```python
from build123d import *

# Parameters (mm, degrees)
SKETCH1_R           = 2.0701
SKETCH1_R_2         = 14.2875
BOSS_EXTRUDE1_DEPTH = 2.286


with BuildPart() as part:
    # Sketch1 → Boss-Extrude1 (new body)
    with BuildSketch(Plane.XY.offset(2.286)):
        with BuildLine():
            Line((-24.282138093, -1.253612903), (-13.20363246, -27.386969147))
            ThreePointArc((-13.20363246, -27.386969147), (-12.827181753, -28.600844397), (-12.7, -29.865373188))
            Line((-12.7, -29.865373188), (-12.7, -65.148356459))
            Line((-12.7, -65.148356459), (-11.173356459, -66.675))
            Line((-11.173356459, -66.675), (11.173356459, -66.675))
            Line((11.173356459, -66.675), (12.7, -65.148356459))
            Line((12.7, -65.148356459), (12.7, -29.865373188))
            ThreePointArc((12.7, -29.865373188), (12.827181753, -28.600844397), (13.20363246, -27.386969147))
            Line((13.20363246, -27.386969147), (24.282138093, -1.253612903))
            Line((24.282138093, -1.253612903), (24.282138093, 0.905387097))
            Line((24.282138093, 0.905387097), (13.596092395, 19.110856459))
            Line((13.596092395, 19.110856459), (12.069448854, 20.6375))
            Line((12.069448854, 20.6375), (-12.069448854, 20.6375))
            Line((-12.069448854, 20.6375), (-13.596092395, 19.110856459))
            Line((-13.596092395, 19.110856459), (-24.282138093, 0.905387097))
            Line((-24.282138093, 0.905387097), (-24.282138093, -1.253612903))
        make_face()
        with Locations((-9.2075, 15.947857811)):
            Circle(SKETCH1_R, mode=Mode.SUBTRACT)
        with Locations((-18.415, 0)):
            Circle(SKETCH1_R, mode=Mode.SUBTRACT)
        with Locations((0, -47.625)):
            Circle(SKETCH1_R, mode=Mode.SUBTRACT)
        with Locations((0, -22.225)):
            Circle(SKETCH1_R, mode=Mode.SUBTRACT)
        Circle(SKETCH1_R_2, mode=Mode.SUBTRACT)
        with Locations((0, -34.925)):
            Circle(SKETCH1_R, mode=Mode.SUBTRACT)
        with Locations((0, -60.325)):
            Circle(SKETCH1_R, mode=Mode.SUBTRACT)
        with Locations((18.415, 0)):
            Circle(SKETCH1_R, mode=Mode.SUBTRACT)
        with Locations((9.2075, 15.947857811)):
            Circle(SKETCH1_R, mode=Mode.SUBTRACT)
    extrude(amount=-BOSS_EXTRUDE1_DEPTH)


solid = part.part
```
CAD build for the part. Positions are in the model's coordinates, mm. A direction names the side the tool comes from. Coordinates: 2 decimals unless noted, no trailing zeros. Order: outer loops, then holes, each group sorted by start corner. A loop starts at its lowest first (then second) coordinate and runs counter-clockwise, first axis right, second up. Notation, with made-up numbers: (43.25, 32) - (90.25, 32) arc R33 cw to (90.25, 63) - close; hole circle Ø4 at (39, -36). An arc over 180 degrees is marked (long way). Answer in a Markdown table with one row per item.
1. 3-axis set-ups, long thin cutter, end or side, ignore diameter. For faces 4 (the face through (-12.7, -47, 1)), 5 (the face through (16.347, 0.091, 1.159)), 6 (the face through (12.7, -48, 1)): which of +Z, -Z, +X, -X, +Y, -Y reach the whole face in a straight line?
Answer:
| item | result |
|---|---|
| face 4 | +Z, -Z, -X, -Y |
| face 5 | +Z, -Z |
| face 6 | +Z, -Z, +X, -Y |
2. Drill centre lines: L1, parallel to Y at x = 0, z = 1.7 (1 decimal); L2, parallel to Y at x = 10, z = 0.8 (1 decimal); L3, parallel to X at y = -54.5, z = 0.7. Where is each one in solid material? Low to high. Write a range as from..to.
Answer:
| item | result |
|---|---|
| L1 | -66.7..-62.4, -58.3..-49.7, -45.6..-37, -32.9..-24.3, -20.2..-14.3, 14.3..20.6 |
| L2 | -66.7..-10.2, 10.2..14, 17.9..20.6 |
| L3 | -12.7..12.7 |
3. Slice it at B-B, the plane x = 0. List the corners of the cut face in (y, z) (1 decimal), then the cut area to 3 significant figures.
Answer:
| item | result |
|---|---|
| outline | (-66.7, 0) - (-62.4, 0) - (-62.4, 2.3) - (-66.7, 2.3) - close; (-58.3, 0) - (-49.7, 0) - (-49.7, 2.3) - (-58.3, 2.3) - close; (-45.6, 0) - (-37, 0) - (-37, 2.3) - (-45.6, 2.3) - close; (-32.9, 0) - (-24.3, 0) - (-24.3, 2.3) - (-32.9, 2.3) - close; (-20.2, 0) - (-14.3, 0) - (-14.3, 2.3) - (-20.2, 2.3) - close; (14.3, 0) - (20.6, 0) - (20.6, 2.3) - (14.3, 2.3) - close |
| area | 96.4 mm² |
4. Flat gauge pins, fed straight in: P1, Ø2.5, axis at x = 0, y = -34.925, coming from the -Z side; P2, Ø0.7, axis at y = -40, z = 0.5, coming from the -X side. Where does each tip first touch, or does it go through?
Answer:
| item | result |
|---|---|
| P1 | through |
| P2 | x = -12.7 |
5. Pull direction Y, two halves, no side cores. Call faces 1 (the face through (8.94, 18, 1.16)), 2 (the face through (24.282, 0, 1)), 3 (the face through (-12.83, -28.58, 1.16)): +Y half, -Y half, draft (parallel to the pull), parting line (faces both ways), or undercut.
Answer:
| item | result |
|---|---|
| face 1 | undercut |
| face 2 | draft |
| face 3 | -Y half |
6. Slice it at D-D, the plane y = -12. List the corners of the cut face in (x, z).
Answer:
| item | result |
|---|---|
| outline | (-19.73, 0) - (-7.75, 0) - (-7.75, 2.29) - (-19.73, 2.29) - close; (7.75, 0) - (19.73, 0) - (19.73, 2.29) - (7.75, 2.29) - close |
7. Slice it at C-C, the plane z = 1.65. Give the number of separate pieces and of enclosed holes in the cut face, then the cut area to 3 significant figures.
Answer:
| item | result |
|---|---|
| separate pieces | 1 |
| enclosed holes | 9 |
| area | 2,060 mm² |
8. Slice it at A-A, the plane y = 0. List the corners of the cut face in (x, z), then the cut area to 3 significant figures.
Answer:
| item | result |
|---|---|
| outline | (-24.28, 0) - (-20.49, 0) - (-20.49, 2.29) - (-24.28, 2.29) - close; (-16.34, 0) - (-14.29, 0) - (-14.29, 2.29) - (-16.34, 2.29) - close; (14.29, 0) - (16.34, 0) - (16.34, 2.29) - (14.29, 2.29) - close; (20.49, 0) - (24.28, 0) - (24.28, 2.29) - (20.49, 2.29) - close |
| area | 26.8 mm² |
